Geometry: see drawing. Coordinates: mm, zero at the bounding-box minimum. A direction names the side the tool comes from. Round coordinates to 2 decimals unless told otherwise and drop trailing zeros. Write each loop counter-clockwise with the first axis right and the second up, starting at its lowest first coordinate (ties: lowest second). Pieces come first, ordered by that corner, then holes. Notation, with made-up numbers: (-10.75, 77) -> (19.25, 77) arc R20 ccw to (19.25, 85) -> close; hole circle Ø5 at (-19.5, 31.25). An arc over 180 degrees is marked (long way). Use CSV: the item, a comma, the result in double quotes.
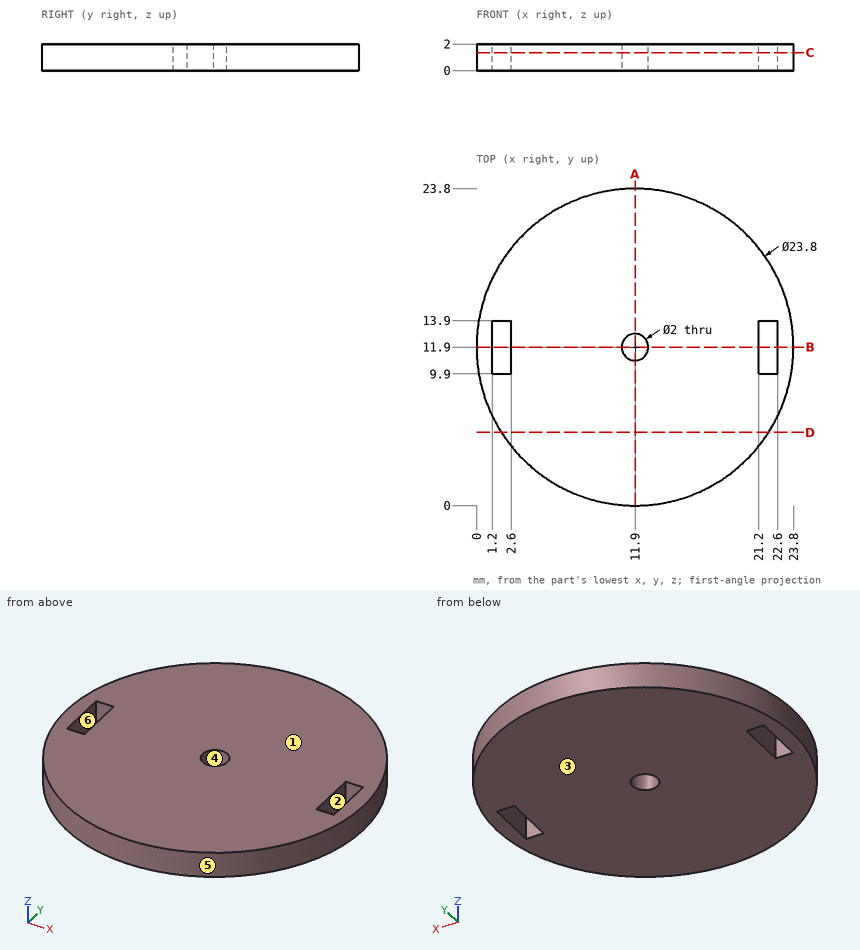
Item 1: Section query B-B on y = 11.9. Return the cut outline in (x, z).
Worked answers:
outline,"(0, 0) -> (1.2, 0) -> (1.2, 2) -> (0, 2) -> close; (2.6, 0) -> (10.9, 0) -> (10.9, 2) -> (2.6, 2) -> close; (12.9, 0) -> (21.2, 0) -> (21.2, 2) -> (12.9, 2) -> close; (22.6, 0) -> (23.8, 0) -> (23.8, 2) -> (22.6, 2) -> close"
Item 2: Pull-direction query (Y, two-part tool) for the marked faces 3, 4, 5 and 6; classes: +Y half, -Y half, draft (parallel to the pull), parting line (faces both ways), or undercut.
Worked answers:
face 3,"draft"
face 4,"undercut"
face 5,"parting line"
face 6,"undercut"
Item 3: First-contact query: pin 1 Ø0.6 at (y, z) = (11.5, 1) entering from +X; pin 2 Ø1.2 at (x, y) = (11.9, 11.9) entering from +Z; pin 3 Ø1.1 at (x, z) = (2, 1.5) entering from +Y; pin 4 Ø1 at (y, z) = (2.5, 1) entering from -X. Flat tips, straight axial feed; report the tip coordinate or a pass-through.
Worked answers:
pin 1,"stops at x = 23.8"
pin 2,"passes through"
pin 3,"stops at y = 19.26"
pin 4,"stops at x = 4"
Item 4: Section query C-C on z = 1.35. Return the cut outline in (x, y), plus the area to 3 significant figures.
Worked answers:
outline,"circle Ø23.8 at (11.9, 11.9); hole (1.2, 9.9) -> (2.6, 9.9) -> (2.6, 13.9) -> (1.2, 13.9) -> close; hole circle Ø2 at (11.9, 11.9); hole (21.2, 9.9) -> (22.6, 9.9) -> (22.6, 13.9) -> (21.2, 13.9) -> close"
area,"431 mm²"
Item 5: Line query: line 1 (Y direction, x = 11.9, z = 1); line 2 (X direction, y = 10, z = 1.2); line 3 (Y direction, x = 15, z = 0.8). Output: solid intervals per line, ascending.
Worked answers:
line 1,"y = 0 to 10.9, 12.9 to 23.8"
line 2,"x = 0.15 to 1.2, 2.6 to 21.2, 22.6 to 23.65"
line 3,"y = 0.41 to 23.39"
Item 6: Set-up query: the marked faces 1 and 2. Return all of +Z, -Z, +X, -X, +Y, -Y with unobstructed straight access to the full face (end or side cutting, diameter ignored); none if empty.
Worked answers:
face 1,"+Z, +X, -X, +Y, -Y"
face 2,"+Z, -Z"
Item 7: Section query A-A on x = 11.9. Return the cut outline in (y, z), plus the area to 3 significant figures.
Worked answers:
outline,"(0, 0) -> (10.9, 0) -> (10.9, 2) -> (0, 2) -> close; (12.9, 0) -> (23.8, 0) -> (23.8, 2) -> (12.9, 2) -> close"
area,"43.6 mm²"
Item 8: Section query D-D on y = 5.5. Return the cut outline in (x, z).
Worked answers:
outline,"(1.87, 0) -> (21.93, 0) -> (21.93, 2) -> (1.87, 2) -> close"
